Autodesk Inventor part; units mm, degrees
ref_plane "YZ Plane" through (0, 0, 0) normal (1, 0, 0) x (0, 1, 0)
ref_plane "XZ Plane" through (0, 0, 0) normal (0, 1, 0) x (-1, 0, 0)
ref_plane "XY Plane" through (0, 0, 0) normal (0, 0, 1) x (1, 0, 0)
sketch "Sketch1" plane through (0, 0, 0) normal (0, 0, 1) x (1, 0, 0)
  circle A0 centre (0, 0) radius 100
  circle A1 centre (0, 0) radius 56
  circle A2 centre (0, 0) radius 67
  circle A3 centre (0, 0) radius 7.5
  dimension "d0" = 200
  dimension "d1" = 112
  dimension "d2" = 11
  dimension "d3" = 15
extrude "Extrusion1" [suppressed]
extrude "Extrusion2" [suppressed]
extrude "Extrusion3" [suppressed]
extrude "Extrusion4" [suppressed]
sketch "Sketch2" plane through (0, 0, 0) normal (1, 0, 0) x (0, 1, 0)
  line L0 (0, 42.5) -> (0, -42.5)
  line L1 (0, 42.5) -> (8.5, 42.5)
  line L2 (8.5, 42.5) -> (8.5, -42.5)
  line L3 (8.5, -42.5) -> (0, -42.5)
  line L4 (56, 31) -> (56, -31)
  line L5 (0, 0) -> (100, 0) construction
  line L6 (56, 31) -> (12.3593, 31)
  line L7 (56, -31) -> (12.3593, -31)
  line L8 (67, 20) -> (67, -20)
  line L9 (100, 25) -> (100, -25)
  line L10 (56, 20) -> (67, 20)
  line L11 (67, -20) -> (56, -20)
  line L12 (100, 25) -> (67, 25)
  line L13 (67, 25) -> (67, 20)
  line L14 (67, -20) -> (67, -25)
  line L15 (67, -25) -> (100, -25)
  line L16 (12.3593, 31) -> (12.3593, 29.5)
  line L17 (12.3593, 29.5) -> (8.5, 29.5)
  line L18 (12.3593, -31) -> (12.3593, -29.5)
  line L19 (12.3593, -29.5) -> (8.5, -29.5)
  point P0 (56, 0)
  point P1 (8.5, 32.5)
  point P2 (8.5, -32.5)
  point P3 (67, 0)
  point P4 (4.25, 42.5)
  dimension "d12" = 85
  dimension "d13" = 8.5
  dimension "d15" = 100
  dimension "d16" = 56
  dimension "d17" = 40
  dimension "d18" = 11
  dimension "d19" = 50
  dimension "d27" = 13
  dimension "d28" = 1.5
revolve "Revolution1" add sketch "Sketch2" angle 360 about axis through (0, 0, 42.5) along (0, 0, -1)
fillet "Fillet1" radius 20 2 edges at (0, -100, 25) (0, -100, -25)
fillet "Fillet2" radius 10 2 edges at (0, -56, 31) (0, -56, -31)
sketch "Sketch3" plane through (0, 0, 42.5) normal (0, 0, 1) x (1, 0, 0)
  circle A0 centre (0, 0) radius 8.5
  line L0 (-6.75, 5.166) -> (-6.75, -5.166)
  line L1 (6.75, 5.166) -> (6.75, -5.166)
  circle A1 centre (0, 0) radius 8.5
  circle A2 centre (0, 0) radius 8.5
  line L2 (-6.75, 0) -> (6.75, 0) construction
  circle A3 centre (0, 3.5) radius 2
  circle A4 centre (0, 0) radius 8.5
  point P0 (6.6019, 3.3672)
  point P1 (6.6019, -3.3672)
  point P2 (0, 5.5)
  point P3 (0, 8.5)
  dimension "d29" = 4
  dimension "d24" = 13.5
  dimension "d30" = 3
extrude "Extrusion5" cut sketch "Sketch3" against normal blind 9 contours A0 L1 | L0 A0
hole "Hole1" at (0, 3.5, 42.5) direction (0, 0, -1) diameter 3.242 depth 10
mirror "Mirror1" about plane through (0, 0, 0) normal (0, 0, 1) of "Extrusion5", "Hole1"
properties part number "motor at24v"
Geometry: final body of the model. Coordinates: model frame, mm. A direction names the side the tool comes from. Give positions to 0.01 mm unless a question says otherwise; leave off trailing zeros. Write each loop counter-clockwise with the first axis right and the second up, starting at its lowest first coordinate (ties: lowest second). Pieces come first, ordered by that corner, then holes.
(1) First-contact query: P1, Ø1, axis at y = -26.5, z = -21, coming from the +X side; P2, Ø3, axis at x = 54.5, y = 27, coming from the +Z side; P3, Ø1.9, axis at x = 0, y = 3.5, coming from the +Z side. Flat tips, straight axial feed; report the tip coordinate or a pass-through.
(2) Mould query, pull axis X, two halves, no side actions, for faces 1 (the flat face through (-54.3, -15.2, -20)), 2 (the flat face through (-65, -18, 25)), 3 (the cylindrical face through (30.04, 95.38, -0.07)), 4 (the flat face through (-6.75, 0, 38)). Classes: released by +X, released by -X, zero draft, split by the parting line, or undercut.
(3) Access query for faces 5 (the cylindrical face through (0.37, -8.49, 34.46)), 6 (the flat face through (-65, -18, -25)), 7 (the flat face through (-6.75, 0, -38)), 8 (the flat face through (6.75, 0, -38)). Directions: +Z, -Z, +X, -X, +Y, -Y. A direction counts if a zero-diameter tool reaches every point of the face in a straight line with its end or side. Return the directions, or none.
(4) Ray query, line 1 (X direction, y = 0, z = 21); line 2 (Z direction, x = -0.5, y = 63.5); line 3 (X direction, y = 0, z = -23.2) (3 decimals). Return the intervals inside material, ascending.
(5) Cut plane A-A, the plane z = 1.5. Return loops of the section in (x, y).
Values follow:
1. P1: stops at x = 88.79
1. P2: stops at z = 20
1. P3: stops at z = 32.5
2. face 1: undercut
2. face 2: zero draft
2. face 3: split by the parting line
2. face 4: released by -X
3. face 5: +Z
3. face 6: -Z
3. face 7: -Z, -X, +Y, -Y
3. face 8: -Z, +X, +Y, -Y
4. line 1: x = -92 to -67, -56 to 56, 67 to 92
4. line 2: z = -20 to 20
4. line 3: x = -88.292 to -67, -55.755 to 55.755, 67 to 88.292
5. outline: circle Ø200 at (0, 0)
